from build123d import *

# Parameters (mm, degrees)
SKETCH_1_R               = 18.5
EXTRUDE_1_DEPTH          = 24
SKETCH_2_R               = 6
EXTRUDE_2_DEPTH          = 6
SKETCH_3_R               = 1.5
CUT_EXTRUDE_1_DEPTH      = 4
SKETCH_4_R               = 3
EXTRUDE_3_DEPTH          = 11.5
CHAMFER_1_SIZE           = 0.1
CUT_EXTRUDE_2_DEPTH      = 7
PATTERN_CIRCULAR_1_COUNT = 6
SKETCH_6_R               = 18
EXTRUDE_4_DEPTH          = 57
SKETCH_7_R               = 6.5
EXTRUDE_5_DEPTH          = 3.5
FILLET_1_R               = 1
SKETCH_8_R               = 1.5
EXTRUDE_6_DEPTH          = 1
SKETCH_9_W               = 0.5
SKETCH_9_H               = 4
EXTRUDE_7_DEPTH          = 8
FILLET_2_R               = 0.5
SKETCH_10_R              = 1
CUT_EXTRUDE_3_DEPTH      = 0.5
SKETCH_11_R              = 1
CUT_EXTRUDE_4_DEPTH      = 0.5
FILLET_3_R               = 0.8


with BuildPart() as part:
    # Sketch 1 → Extrude 1 (new body)
    with BuildSketch(Plane.XY):
        Circle(SKETCH_1_R)
    extrude(amount=EXTRUDE_1_DEPTH)

    # Sketch 2 → Extrude 2 (add)
    with BuildSketch(Plane.XY.offset(24)):
        with Locations((0, 7)):
            Circle(SKETCH_2_R)
    extrude(amount=EXTRUDE_2_DEPTH)

    # Sketch 3 → Cut-Extrude 1 (cut)
    with BuildSketch(Plane.XY.offset(24)):
        with Locations((15.5, 0)):
            Circle(SKETCH_3_R)
    cut_extrude_1 = extrude(amount=-CUT_EXTRUDE_1_DEPTH, mode=Mode.SUBTRACT)

    # Sketch 4 → Extrude 3 (add)
    with BuildSketch(Plane.XY.offset(30)):
        with Locations((0, 7)):
            Circle(SKETCH_4_R)
    extrude(amount=EXTRUDE_3_DEPTH)

    # Chamfer 1
    chamfer_1_edges = [part.edges().sort_by_distance(p)[0] for p in [
        (-3, 7, 41.5),
    ]]
    chamfer(chamfer_1_edges, length=CHAMFER_1_SIZE)

    # Sketch 5 → Cut-Extrude 2 (cut)
    with BuildSketch(Plane.XY.offset(41.5)):
        with BuildLine():
            Line((-2.589731968, 5.485639298), (2.589731968, 5.485639298))
            ThreePointArc((2.589731968, 5.485639298), (0, 4), (-2.589731968, 5.485639298))
        make_face()
    extrude(amount=-CUT_EXTRUDE_2_DEPTH, mode=Mode.SUBTRACT)

    # Pattern Circular 1: Cut-Extrude 1 ×6 about axis
    pattern_circular_1_axis = Axis((0, 0, 0), (0, 0, 1))
    for i in range(1, PATTERN_CIRCULAR_1_COUNT):
        add(cut_extrude_1.rotate(pattern_circular_1_axis, i * 360 / PATTERN_CIRCULAR_1_COUNT), mode=Mode.SUBTRACT)

    # Sketch 6 → Extrude 4 (add)
    with BuildSketch(Plane(origin=(0, 0, 0), x_dir=(-1, 0, 0), z_dir=(0, 0, -1))):
        Circle(SKETCH_6_R)
    extrude(amount=EXTRUDE_4_DEPTH)

    # Sketch 7 → Extrude 5 (add)
    with BuildSketch(Plane(origin=(0, 0, -57), x_dir=(-1, 0, 0), z_dir=(0, 0, -1))):
        Circle(SKETCH_7_R)
    extrude(amount=EXTRUDE_5_DEPTH)

    # Fillet 1
    fillet_1_edges = [part.edges().sort_by_distance(p)[0] for p in [
        (6.5, 0, -60.5),
    ]]
    fillet(fillet_1_edges, radius=FILLET_1_R)

    # Sketch 8 → Extrude 6 (add)
    with BuildSketch(Plane(origin=(0, 0, -60.5), x_dir=(-1, 0, 0), z_dir=(0, 0, -1))):
        Circle(SKETCH_8_R)
    extrude(amount=EXTRUDE_6_DEPTH)

    # Sketch 9 → Extrude 7 (add)
    with BuildSketch(Plane(origin=(0, 0, -57), x_dir=(-1, 0, 0), z_dir=(0, 0, -1))):
        with Locations((14.25, 0)):
            Rectangle(SKETCH_9_W, SKETCH_9_H)
        with Locations((-14.25, 0)):
            Rectangle(SKETCH_9_W, SKETCH_9_H)
    extrude(amount=EXTRUDE_7_DEPTH)

    # Fillet 2
    fillet_2_edges = [part.edges().sort_by_distance(p)[0] for p in [
        (-14.25, -2, -65),
        (-14.25, 2, -65),
        (14.25, 2, -65),
        (14.25, -2, -65),
    ]]
    fillet(fillet_2_edges, radius=FILLET_2_R)

    # Sketch 10 → Cut-Extrude 3 (cut)
    with BuildSketch(Plane.ZY.offset(14.5)):
        with Locations((-62.5, 0)):
            Circle(SKETCH_10_R)
    extrude(amount=-CUT_EXTRUDE_3_DEPTH, mode=Mode.SUBTRACT)

    # Sketch 11 → Cut-Extrude 4 (cut)
    with BuildSketch(Plane(origin=(14.5, 0, 0), x_dir=(0, 0, -1), z_dir=(1, 0, 0))):
        with Locations((62.5, 0)):
            Circle(SKETCH_11_R)
    extrude(amount=-CUT_EXTRUDE_4_DEPTH, mode=Mode.SUBTRACT)

    # Fillet 3
    fillet_3_edges = [part.edges().sort_by_distance(p)[0] for p in [
        (1.5, 0, -61.5),
    ]]
    fillet(fillet_3_edges, radius=FILLET_3_R)


solid = part.part
Can you work these out from the model? Positions are in its coordinate system, mm. A direction names the side the tool comes from. Give positions to 0.01 mm unless a question says otherwise; leave off trailing zeros. Write each loop counter-clockwise with the first axis right and the second up, starting at its lowest first coordinate (ties: lowest second). Pieces come first, ordered by that corner, then holes. Notation, with made-up numbers: M 11.5,27 L 29.5,27 A30 cw 29.5,60 Z; hole C -21,-21.5 d4. An arc over 180 degrees is marked long. Answer in a Markdown table with one row per item. Add a question column.
Item 1: Imagine slicing it at D-D, the plane z = 12.5. Write out the boundary of the cut face in (x, y).
Item 2: On a 3-axis mill with a long thin cutter (end or side, diameter ignored), from which of +Z, -Z, +X, -X, +Y, -Y can I reach the whole of each face in a straight line? I mean faces 1 (the flat face through (14.5, 0, -61)), 2 (the flat face through (-14, 0, -61)), 3 (the cylindrical face through (-0.78, 12.95, 26.96)). Say none if no direction works.
Item 3: Imagine slicing it at C-C, the plane z = -48. Write out the boundary of the cut face in (x, y), plus the area to 3 significant figures.
Item 4: For pin 1 Ø2.5 at (x, y) = (-7.75, 13.42) entering from -Z; pin 2 Ø9 at (x, y) = (-2, -1.5) entering from -Z; pin 3 Ø1.5 at (x, z) = (14, -16) entering from +Y, each with a flat end and sliding along its axis, tell me the tip position at first contact or that it passes through.
Item 5: We'd pull the mould along Y, two halves only. Please class faces 4 (the cylindrical face through (-4.01, -18.06, 11.83)), 5 (the flat face through (8, -13, 20)), 6 (the flat face through (0, -8, -57)): released by +Y, released by -Y, zero draft, split by the parting line, or undercut.
Item 6: Imagine slicing it at B-B, the plane y = -8. Write out the boundary of the cut face in (x, z).
Item 7: Imagine slicing it at A-A, the plane x = 12. Write out the boundary of the cut face in (y, z).
Item 8: Please list where these lines run through material, in increasing order: L1, parallel to Y at x = -7, z = 21; L2, parallel to Y at x = -7.75, z = 22.3; L3, parallel to Z at x = -12, y = 12.5.
Evaluation:
| question | item | result |
|---|---|---|
| 1 | outline | C 0,0 d37 |
| 2 | face 1 | -Z, +X, +Y, -Y |
| 2 | face 2 | -Z, +Y, -Y |
| 2 | face 3 | +Z |
| 3 | outline | C 0,0 d36 |
| 3 | area | 1,020 mm² |
| 4 | pin 1 | stops at z = -57 |
| 4 | pin 2 | stops at z = -61.5 |
| 4 | pin 3 | stops at y = 12.18 |
| 5 | face 4 | split by the parting line |
| 5 | face 5 | undercut |
| 5 | face 6 | zero draft |
| 6 | outline | M -16.68,0 L -16.12,0 L -16.12,-57 L 16.12,-57 L 16.12,0 L 16.68,0 L 16.68,24 L -16.68,24 Z |
| 7 | outline | M -14.08,0 L -13.42,0 L -13.42,-57 L 13.42,-57 L 13.42,0 L 14.08,0 L 14.08,24 L -14.08,24 Z |
| 8 | L1 | y = -17.12 to -14.72, -12.12 to 12.12, 14.72 to 17.12 |
| 8 | L2 | y = -16.8 to -14.92, -11.92 to 11.92, 14.92 to 16.8 |
| 8 | L3 | z = -57 to 24 |
